Verification items for the finished model (mm, model axes). A direction names the side the tool comes from. Coordinates: 2 decimals unless noted, no trailing zeros. Loops run counter-clockwise (first coordinate to the right, second up) from the corner with the lowest first, then second, coordinate; pieces in that order, holes last. Notation, with made-up numbers: (16, -9.5) - (24, -9.5) arc R26 ccw to (24, 4.5) - close; hole circle Ø2 at (23.5, 12). An arc over 180 degrees is marked (long way). One line per item, written item: value. Start each with the question number.
(1) Section check D-D (y = -2.5). Record the boundary of the cut face in (x, z) (3 decimals), plus the area to 3 significant figures.
(2) Section check A-A (x = -18). Record the boundary of the cut face in (y, z) (3 decimals), plus the area to 3 significant figures.
(3) Gauge pin test, flat ends, axial feed: P1, Ø5, axis at x = 4, z = -2.5, coming from the +Y side; P2, Ø10, axis at x = 12.5, y = -21.5, coming from the -Z side; P3, Ø4, axis at y = -16.5, z = -5.5, coming from the -X side; P4, Ø6, axis at y = -36, z = 0.5, coming from the -X side. Record the tip position at first contact, or that the pin passes through.
(4) Set-up check for faces 1 (the face through (11, -21, 0)), 2 (the face through (23, -1, -5)), 3 (the face through (-15, -21, 0)): record each of +Z, -Z, +X, -X, +Y, -Y from which the full face is reachable in a straight line by a thin tool's end or side.
(5) Draft check along X on faces 4 (the face through (15.727, -17.418, 1.409)), 5 (the face through (-20.4, -20.28, 2.21)), 6 (the face through (20.43, -20.28, 2.18)). Enter one of: +X half, -X half, draft (parallel to the pull), parting line (faces both ways), or undercut.
(6) Thickness scan on probe 1 along Y at (x, z) = (16, 1.7); probe 2 along Y at (x, z) = (6, 1.1); probe 3 along Z at (x, y) = (-18, -2.1) (3 decimals). Record the ranges inside material, lowest first. Write a range as [from, to].
(7) Section check C-C (y = -19.5). Record the boundary of the cut face in (x, z), plus the area to 3 significant figures.
(8) Section check B-B (z = -5). Record the boundary of the cut face in (x, y) (3 decimals), plus the area to 4 significant figures.
```python
from build123d import *

# Parameters (mm, degrees)
F1_DEPTH      = 3
F2_R          = 2.875
F3_DEPTH      = 25
F4_W          = 10
F4_H          = 10
F5_DEPTH      = 37
F5_DEPTH_BACK = 3
F7_DEPTH      = 25
F8_R          = 2.1
F9_DEPTH      = 25


with BuildPart() as f1:
    # F0 (on Front) → F1 (new body)
    with BuildSketch(Plane.XZ):
        with BuildLine():
            Line((21, 0), (-21, 0))
            ThreePointArc((-21, 0), (-22.414214, -0.585786), (-23, -2))
            Line((-23, -2), (-23, -8))
            ThreePointArc((-23, -8), (-22.414214, -9.414214), (-21, -10))
            Line((-21, -10), (21, -10))
            ThreePointArc((21, -10), (22.414214, -9.414214), (23, -8))
            Line((23, -8), (23, -2))
            ThreePointArc((23, -2), (22.414214, -0.585786), (21, 0))
        make_face()
    extrude(amount=F1_DEPTH)

    # F2 (on face) → F3 (cut)
    with BuildSketch(Plane.XZ.offset(3)):
        with Locations((-18, -5)):
            Circle(F2_R)
        with Locations((18, -5)):
            Circle(F2_R)
    extrude(amount=-F3_DEPTH, mode=Mode.SUBTRACT)

    # F4 (on face) → F5 (join, two sides)
    with BuildSketch(Plane.XZ.offset(3)) as f5_sk:
        with BuildLine():
            Line((-21, 0.779364), (-21, 0))
            Line((-21, 0), (-9, 0))
            Line((-9, 0), (1, 0))
            Line((1, 0), (21, 0))
            Line((21, 0), (21, 0.779364))
            ThreePointArc((21, 0.779364), (20.414214, 2.193577), (19, 2.779364))
            Line((19, 2.779364), (-19, 2.779364))
            ThreePointArc((-19, 2.779364), (-20.414214, 2.193577), (-21, 0.779364))
        make_face()
        with Locations((-4, -5)):
            Rectangle(F4_W, F4_H)
    extrude(amount=F5_DEPTH)
    extrude(f5_sk.sketch, amount=-F5_DEPTH_BACK)

    # F6 (on face) → F7 (cut)
    with BuildSketch(Plane.YZ.offset(1)):
        Polygon((-3, -10), (-40, 0), (-40, -10), align=None)
    extrude(amount=-F7_DEPTH, mode=Mode.SUBTRACT)

    # F8 (on face) → F9 (cut)
    with BuildSketch(Plane.XY.offset(2.779364)):
        with Locations((16, -19.5)):
            Circle(F8_R)
        with Locations((6, -24.5)):
            Circle(F8_R)
    extrude(amount=-F9_DEPTH, mode=Mode.SUBTRACT)


solid = f1.part
```
Responses:
1. outline: (-23, -8) arc R2 ccw to (-21, -10) - (21, -10) arc R2 ccw to (23, -8) - (23, -2) arc R2 ccw to (21, 0) - (21, 0.779) arc R2 ccw to (19, 2.779) - (-19, 2.779) arc R2 ccw to (-21, 0.779) - (-21, 0) arc R2 ccw to (-23, -2) - close; hole circle Ø5.75 at (-18, -5); hole circle Ø5.75 at (18, -5)
1. area: 520 mm²
2. outline: (-40, 0) - (-3, 0) - (-3, -2.125) - (0, -2.125) - (0, 2.779) - (-40, 2.779) - close; (-3, -10) - (0, -10) - (0, -7.875) - (-3, -7.875) - close
2. area: 124 mm²
3. P1: stops at y = 0
3. P2: stops at z = 0
3. P3: stops at x = -9
3. P4: stops at x = -21
4. face 1: -Z, +X, -Y
4. face 2: +Z, -Z, +X, +Y, -Y
4. face 3: -Z, -X, -Y
5. face 4: undercut
5. face 5: -X half
5. face 6: +X half
6. probe 1: y = [-40, -21.6], [-17.4, 0]
6. probe 2: y = [-40, -26.6], [-22.4, 0]
6. probe 3: z = [-10, -7.875], [-2.125, 2.779]
7. outline: (-21, 0) - (-9, 0) - (-9, -5.54) - (1, -5.54) - (1, 0) - (13.9, 0) - (13.9, 2.78) - (-19, 2.78) arc R2 ccw to (-21, 0.78) - close; (18.1, 0) - (21, 0) - (21, 0.78) arc R2 ccw to (19, 2.78) - (18.1, 2.78) - close
7. area: 159 mm²
8. outline: (-23, -3) - (-20.875, -3) - (-20.875, 0) - (-23, 0) - close; (-15.125, -3) - (-9, -3) - (-9, -21.5) - (1, -21.5) - (1, -3) - (15.125, -3) - (15.125, 0) - (-15.125, 0) - close; (20.875, -3) - (23, -3) - (23, 0) - (20.875, 0) - close
8. area: 288.5 mm²
